```python
from build123d import *

# Parameters (mm, degrees)
F0_W     = 60.833
F0_H     = 111.7092
F1_DEPTH = 5.08
F2_W     = 5.094256
F2_H     = 16.649162
F3_DEPTH = 7.62


with BuildPart() as f1:
    # F0 (on Front) → F1 (new body)
    with BuildSketch(Plane.XZ):
        with Locations((2.253074, 0)):
            Rectangle(F0_W, F0_H)
    extrude(amount=-F1_DEPTH)

    # F2 (on face) → F3 (join)
    with BuildSketch(Plane(origin=(0, 5.08, 0), x_dir=(-1, 0, 0), z_dir=(0, 1, 0))):
        with Locations((-24.730271, 0)):
            Rectangle(F2_W, F2_H)
    extrude(amount=-F3_DEPTH)


solid = f1.part
```
Model file for the job. Use its own axes, mm. A direction names the side the tool comes from. Coordinates: 2 decimals unless noted, no trailing zeros. Loops run counter-clockwise (first coordinate to the right, second up) from the corner with the lowest first, then second, coordinate; pieces in that order, holes last. Notation, with made-up numbers: (76.25, -13) - (120.25, -13) arc R30 cw to (120.25, 12) - close; hole circle Ø11 at (-39.75, -39). An arc over 180 degrees is marked (long way). Answer as a JSON object with one key per item and string values. Group by question number.
(1) Cut at B-B (x = 24). Give the cut face in (y, z), then the cut area to 3 significant figures.
(2) Flat gauge pins, fed straight in: pin 1 (1.3 mm diameter, centred on x = 24.5, y = -1, fed in from -Z); pin 2 (3 mm diameter, centred on x = 25, y = -2, fed in from +Z); pin 3 (3 mm diameter, centred on x = -6.5, z = 30, fed in from -Y). Where does each tip first touch, or does it go through?
(3) Cut at A-A (z = 5.5). Give the cut face in (x, y), then the cut area to 3 significant figures.
(4) Probe line 1 along Y through (x, z) = (14.5, 28); line 2 along X through (y, z) = (-2, 7). List the from-to ranges inside material, lowest first.
(5) Cut at C-C (y = -1.25). Give the cut face in (x, z), then the cut area to 3 significant figures.
(6) Tool access for faces 1 (the face through (25, -1, 8.325)), 2 (the face through (22.183, -1, 0)), 3 (the face through (25, -1, -8.325)), 4 (the face through (27.277, -1, 0)): list every direction of +Z, -Z, +X, -X, +Y, -Y with a clear straight run to the whole face (end or side of a thin tool).
(7) Cut at D-D (z = 17.5). Give the cut face in (x, y).
Geometry says:
{
 "1": {"outline": "(-2.54, -8.32) - (0, -8.32) - (0, -55.85) - (5.08, -55.85) - (5.08, 55.85) - (0, 55.85) - (0, 8.32) - (-2.54, 8.32) - close", "area": "610 mm^2"},
 "2": {"pin 1": "stops at z = -8.32", "pin 2": "stops at z = 8.32", "pin 3": "stops at y = 0"},
 "3": {"outline": "(-28.16, 0) - (22.18, 0) - (22.18, -2.54) - (27.28, -2.54) - (27.28, 0) - (32.67, 0) - (32.67, 5.08) - (-28.16, 5.08) - close", "area": "322 mm^2"},
 "4": {"line 1": "y = 0 to 5.08", "line 2": "x = 22.18 to 27.28"},
 "5": {"outline": "(22.18, -8.32) - (27.28, -8.32) - (27.28, 8.32) - (22.18, 8.32) - close", "area": "84.8 mm^2"},
 "6": {"face 1": "+Z, +X, -X, -Y", "face 2": "+Z, -Z, -X, -Y", "face 3": "-Z, +X, -X, -Y", "face 4": "+Z, -Z, +X, -Y"},
 "7": {"outline": "(-28.16, 0) - (32.67, 0) - (32.67, 5.08) - (-28.16, 5.08) - close"}
}
